```python
from build123d import *

# Parameters (mm, degrees)
SKETCH_1_R      = 1.5
EXTRUDE_1_DEPTH = 1.5


with BuildPart() as part:
    # 草图1 → 凸台-拉伸1 (new body)
    with BuildSketch(Plane.XY):
        with BuildLine():
            Line((-15.25, 18), (15.25, 18))
            ThreePointArc((15.25, 18), (17.194543648, 17.194543648), (18, 15.25))
            Line((18, 15.25), (18, -15.25))
            ThreePointArc((18, -15.25), (17.194543648, -17.194543648), (15.25, -18))
            Line((15.25, -18), (-15.25, -18))
            ThreePointArc((-15.25, -18), (-17.194543648, -17.194543648), (-18, -15.25))
            Line((-18, -15.25), (-18, 15.25))
            ThreePointArc((-18, 15.25), (-17.194543648, 17.194543648), (-15.25, 18))
        make_face()
        with Locations((-15.25, 15.25)):
            Circle(SKETCH_1_R, mode=Mode.SUBTRACT)
        with Locations(Location((15.25, 15.25, 0), (0, 0, 180))):
            Circle(SKETCH_1_R, mode=Mode.SUBTRACT)
        with Locations((15.25, -15.25)):
            Circle(SKETCH_1_R, mode=Mode.SUBTRACT)
        with Locations(Location((-15.25, -15.25, 0), (0, 0, 180))):
            Circle(SKETCH_1_R, mode=Mode.SUBTRACT)
    extrude(amount=EXTRUDE_1_DEPTH)


solid = part.part
```
Input: part model. Units: mm. Frame: model coordinates. Give positions to 0.01 mm unless a question says otherwise; leave off trailing zeros. Write each loop counter-clockwise with the first axis right and the second up, starting at its lowest first coordinate (ties: lowest second). Pieces come first, ordered by that corner, then holes. Notation, with made-up numbers: (20.5, 12.25) - (50.5, 12.25) arc R13 ccw to (50.5, 21.25) - close; hole circle Ø3 at (-38, 15). An arc over 180 degrees is marked (long way). Write item = value, one per line. Start each with the question number.
1) Pin query (flat end, axial travel): pin 1 (2.5 mm diameter, centred on x = -15.25, y = 15.25, fed in from -Z); pin 2 (3.5 mm diameter, centred on x = -15.25, y = -15.25, fed in from +Z). Return the tip coordinate at first contact, or that it passes through.
2) Draft query along Y for faces 1 (the face through (0, 0, 1.5)), 2 (the face through (16.75, 15.18, 0.74)), 3 (the face through (17.17, 17.22, 0.74)). Return one class per face: pulls with the +Y half, pulls with the -Y half, needs draft (parallel to the pull), parting line crosses it, or undercut.
3) Cut plane A-A (z = 0.75). Return loops of the section in (x, y), and give its area (3 significant figures).
4) Material intervals for L1, parallel to Y at x = 15.25, z = 0.55; L2, parallel to X at y = 16.5, z = 0.9, sorted ascending. Write a range as [from, to].
Answers follow:
q1.pin_1 = through
q1.pin_2 = 1.5
q2.face_1 = needs draft
q2.face_2 = undercut
q2.face_3 = pulls with the +Y half
q3.outline = (-18, -15.25) arc R2.75 ccw to (-15.25, -18) - (15.25, -18) arc R2.75 ccw to (18, -15.25) - (18, 15.25) arc R2.75 ccw to (15.25, 18) - (-15.25, 18) arc R2.75 ccw to (-18, 15.25) - close; hole circle Ø3 at (-15.25, -15.25); hole circle Ø3 at (-15.25, 15.25); hole circle Ø3 at (15.25, -15.25); hole circle Ø3 at (15.25, 15.25)
q3.area = 1,260 mm^2
q4.L1 = [-18, -16.75], [-13.75, 13.75], [16.75, 18]
q4.L2 = [-17.7, -16.08], [-14.42, 14.42], [16.08, 17.7]
